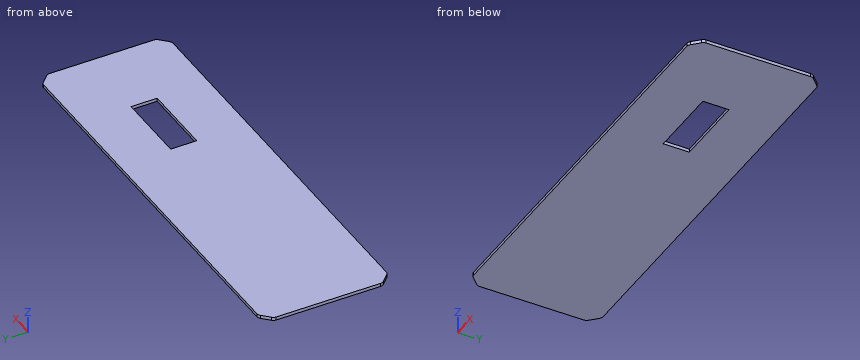
```python
from build123d import *

# Parameters (mm, degrees)
SKETCH1_W           = 400
SKETCH1_H           = 125
BOSS_EXTRUDE1_DEPTH = 3.175
SKETCH2_W           = 69.83
SKETCH2_H           = 25.23
CUT_EXTRUDE1_DEPTH  = 3.175
CHAMFER1_SIZE       = 10
FILLET1_R           = 5


with BuildPart() as part:
    # Sketch1 → Boss-Extrude1 (new body)
    with BuildSketch(Plane.XY):
        Rectangle(SKETCH1_W, SKETCH1_H)
    extrude(amount=BOSS_EXTRUDE1_DEPTH)

    # Sketch2 → Cut-Extrude1 (cut)
    with BuildSketch(Plane.XY.offset(3.175)):
        with Locations((90.085, 0)):
            Rectangle(SKETCH2_W, SKETCH2_H)
    extrude(amount=-CUT_EXTRUDE1_DEPTH, mode=Mode.SUBTRACT)

    # Chamfer1
    chamfer1_edges = [part.edges().sort_by_distance(p)[0] for p in [
        (200, -62.5, 1.5875),
        (-200, -62.5, 1.5875),
        (-200, 62.5, 1.5875),
        (200, 62.5, 1.5875),
    ]]
    chamfer(chamfer1_edges, length=CHAMFER1_SIZE)

    # Fillet1
    fillet1_edges = [part.edges().sort_by_distance(p)[0] for p in [
        (200, 52.5, 1.5875),
        (200, -52.5, 1.5875),
        (-190, -62.5, 1.5875),
        (190, -62.5, 1.5875),
        (-190, 62.5, 1.5875),
        (190, 62.5, 1.5875),
        (-200, -52.5, 1.5875),
        (-200, 52.5, 1.5875),
    ]]
    fillet(fillet1_edges, radius=FILLET1_R)


solid = part.part
```
Geometry: final body of the model. Coordinates: model frame, mm. Round coordinates to 2 decimals unless told otherwise and drop trailing zeros. Order: outer loops, then holes, each group sorted by start corner. A loop starts at its lowest first (then second) coordinate and runs counter-clockwise, first axis right, second up. Notation, with made-up numbers: (0, 86.25) -> (6, 86.25) arc R23 ccw to (6, 98.25) -> close; hole circle Ø3 at (69, 58). An arc over 180 degrees is marked (long way). Use one line per item in the form item = value.
(1) Section B-B on y = -7. Return loops of the section in (x, z) (3 decimals).
Results list:
outline = (-200, 0) -> (55.17, 0) -> (55.17, 3.175) -> (-200, 3.175) -> close; (125, 0) -> (200, 0) -> (200, 3.175) -> (125, 3.175) -> close
(2) Section C-C on z = 1.9. Return loops of the section in (x, y) (3 decimals), and give its area (3 significant figures).
Results list:
outline = (-200, -50.429) arc R5 ccw to (-198.536, -53.964) -> (-191.464, -61.036) arc R5 ccw to (-187.929, -62.5) -> (187.929, -62.5) arc R5 ccw to (191.464, -61.036) -> (198.536, -53.964) arc R5 ccw to (200, -50.429) -> (200, 50.429) arc R5 ccw to (198.536, 53.964) -> (191.464, 61.036) arc R5 ccw to (187.929, 62.5) -> (-187.929, 62.5) arc R5 ccw to (-191.464, 61.036) -> (-198.536, 53.964) arc R5 ccw to (-200, 50.429) -> close; hole (55.17, -12.615) -> (125, -12.615) -> (125, 12.615) -> (55.17, 12.615) -> close
area = 48,000 mm^2
(3) First-contact query: pin 1 Ø1 at (x, y) = (129, 8.5) entering from -Z. Flat tip, straight axial feed; report the tip coordinate or a pass-through.
Results list:
pin_1 = 0
(4) Section A-A on x = 66.5. Return loops of the section in (y, z) (3 decimals), and give its area (3 significant figures).
Results list:
outline = (-62.5, 0) -> (-12.615, 0) -> (-12.615, 3.175) -> (-62.5, 3.175) -> close; (12.615, 0) -> (62.5, 0) -> (62.5, 3.175) -> (12.615, 3.175) -> close
area = 317 mm^2
(5) Ray query, probe 1 along Y at (x, z) = (56, 0.35) (3 decimals); probe 2 along X at (y, z) = (-10, 2.2). Return the intervals inside material, ascending. Write a range as [from, to].
Results list:
probe_1 = [-62.5, -12.615], [12.615, 62.5]
probe_2 = [-200, 55.17], [125, 200]
